```python
from build123d import *

# Parameters (mm, degrees)
SKETCH1_W           = 33.866666666
SKETCH1_H           = 25.4
BOSS_EXTRUDE1_DEPTH = 4.800000052
SKETCH3_W           = 16.333333517
SKETCH3_H           = 16.933333333
CUT_EXTRUDE1_DEPTH  = 99.901754472
SKETCH4_OUTSIDE_W   = 44.386
SKETCH4_OUTSIDE_H   = 35.92
CUT_EXTRUDE3_DEPTH  = 99.901754472
CUT_EXTRUDE4_DEPTH  = 97.639789204


with BuildPart() as part:
    # Sketch1 → Boss-Extrude1 (new body)
    with BuildSketch(Plane(origin=(0, 0, 0), x_dir=(1, 0, 0), z_dir=(0, 1, 0))):
        with Locations((-75.043974065, -23.337368951)):
            Rectangle(SKETCH1_W, SKETCH1_H)
    extrude(amount=BOSS_EXTRUDE1_DEPTH)

    # Sketch3 → Cut-Extrude1 (cut, through all)
    with BuildSketch(Plane(origin=(0, 4.800000052, 0), x_dir=(1, 0, 0), z_dir=(0, 1, 0))):
        with Locations((-83.81064064, -27.570702285)):
            Rectangle(SKETCH3_W, SKETCH3_H)
    extrude(amount=-CUT_EXTRUDE1_DEPTH, mode=Mode.SUBTRACT)

    # Sketch4 outside → Cut-Extrude3 (cut, through all)
    with BuildSketch(Plane(origin=(0, 4.800000052, 0), x_dir=(1, 0, 0), z_dir=(0, 1, 0))):
        with Locations((-75.044, -23.337)):
            Rectangle(SKETCH4_OUTSIDE_W, SKETCH4_OUTSIDE_H)
        Polygon((-91.977307398, -19.104035618), (-75.643973881, -19.104035618), (-75.643973881, -29.264035618), (-58.110640732, -29.264035618), (-58.110640732, -10.637368951), (-91.977307398, -10.637368951), align=None, mode=Mode.SUBTRACT)
    extrude(amount=-CUT_EXTRUDE3_DEPTH, mode=Mode.SUBTRACT)

    # Sketch5 → Cut-Extrude4 (cut, through all)
    with BuildSketch(Plane.XZ):
        Polygon((-91.977307398, 10.637368951), (-83.510640732, 10.637368951), (-83.510640732, 16.093970394), (-83.510640732, 19.104035618), (-91.977307398, 19.104035618), align=None)
    extrude(amount=-CUT_EXTRUDE4_DEPTH, mode=Mode.SUBTRACT)


solid = part.part
```
Model file for the job. Use its own axes, mm. A direction names the side the tool comes from. Round coordinates to 2 decimals unless told otherwise and drop trailing zeros. Write each loop counter-clockwise with the first axis right and the second up, starting at its lowest first coordinate (ties: lowest second). Pieces come first, ordered by that corner, then holes. Notation, with made-up numbers: (-24, 55.5) - (-11, 55.5) arc R26 cw to (-11, 74.5) - close; hole circle Ø1 at (62.5, -2.5). An arc over 180 degrees is marked (long way). One line per item, written item: value.
(1) 3-axis set-ups, long thin cutter, end or side, ignore diameter. For faces 1 (the flat face through (-75.644, 2, 24)), 2 (the flat face through (-83.511, 2, 15)): which of +Z, -Z, +X, -X, +Y, -Y reach the whole face in a straight line?
Values follow:
face 1: +Z, -X, +Y, -Y
face 2: +Z, -Z, -X, +Y, -Y
(2) Cut at C-C, the plane z = 26. Give the cut face in (x, y).
Values follow:
outline: (-75.64, 0) - (-58.11, 0) - (-58.11, 4.8) - (-75.64, 4.8) - close
(3) Wall check: probe 1 along X at (y, z) = (3.3, 21.25); probe 2 along Z at (x, y) = (-77, 3.6). Give the ranges that are in metal, low to high.
Values follow:
probe 1: x = -75.64 to -58.11
probe 2: z = 10.64 to 19.1
(4) Drop a flat-ended pin along its axis: P1, Ø1.4, axis at y = 2.5, z = 24, coming from the -X side. Give the stop position or say it passes through.
Values follow:
P1: stops at x = -75.64
(5) Cut at A-A, the plane y = 1.95. Give the cut face in (x, z).
Values follow:
outline: (-83.51, 10.64) - (-58.11, 10.64) - (-58.11, 29.26) - (-75.64, 29.26) - (-75.64, 19.1) - (-83.51, 19.1) - close
(6) Cut at B-B, the plane x = -76.75. Give the cut face in (y, z).
Values follow:
outline: (0, 10.64) - (4.8, 10.64) - (4.8, 19.1) - (0, 19.1) - close
